Source: CAD feature listing. Evaluate the final solid. Frame: model axes, mm. Round coordinates to 2 decimals unless told otherwise and drop trailing zeros. Order: outer loops, then holes, each group sorted by start corner. A loop starts at its lowest first (then second) coordinate and runs counter-clockwise, first axis right, second up. Notation, with made-up numbers: (45.5, 76.25) - (49.5, 76.25) arc R21 ccw to (49.5, 109.25) - close; hole circle Ø10 at (1.25, 3). An arc over 180 degrees is marked (long way). Put each result on its own line as item: value. Start each with the question number.
1) Section A-A on z = 0. Output: boundary loops of the cut face in (x, y), then the cut area to 3 significant figures.
2) Line query: probe 1 along X at (y, z) = (9, 0); probe 2 along X at (y, z) = (17.75, 3); probe 3 along Z at (x, y) = (30.5, 2). Output: solid intervals per line, ascending. Write a range as [from, to].
3) Mould query, pull axis Z, two halves, no side actions, for faces 1 (the face through (46.99, 12.1, -22.15)), 2 (the face through (-4.88, 10.14, -1.08)), 3 (the face through (50, 12, 0)), 4 (the face through (-1, 12, 25)). Classes: +Z half, -Z half, draft (parallel to the pull), parting line (faces both ways), or undercut.
4) Section C-C on y = 11.25. Output: boundary loops of the cut face in (x, z), then the cut area to 3 significant figures.
5) Section B-B on x = 0. Output: boundary loops of the cut face in (y, z).
6) Contact query for a flat-ended pin moving along its axis: P1, Ø6, axis at x = 0, z = 0, coming from the +Y side. Output: stop coordinate, or through.
```python
from build123d import *

# Parameters (mm, degrees)
SKETCH1_W           = 100
SKETCH1_H           = 50
BOSS_EXTRUDE1_DEPTH = 20
SKETCH2_R           = 15
CUT_EXTRUDE1_DEPTH  = 20
FILLET1_R           = 10
CHAMFER1_SIZE       = 1
MOVE_FACE1_BY       = 10
FILLET2_R           = 5


with BuildPart() as part:
    # Sketch1 → Boss-Extrude1 (new body)
    with BuildSketch(Plane(origin=(0, 0, 0), x_dir=(1, 0, 0), z_dir=(0, 1, 0))):
        Rectangle(SKETCH1_W, SKETCH1_H)
    extrude(amount=BOSS_EXTRUDE1_DEPTH)

    # Sketch2 → Cut-Extrude1 (cut)
    with BuildSketch(Plane(origin=(0, 20, 0), x_dir=(1, 0, 0), z_dir=(0, 1, 0))):
        with Locations(Location((0, 0, 0), (0, 0, 270))):
            Circle(SKETCH2_R)
    extrude(amount=-CUT_EXTRUDE1_DEPTH, mode=Mode.SUBTRACT)

    # Fillet1
    fillet1_edges = [part.edges().sort_by_distance(p)[0] for p in [
        (50, 10, 25),
        (-50, 10, 25),
        (50, 10, -25),
    ]]
    fillet(fillet1_edges, radius=FILLET1_R)

    # Chamfer1
    chamfer1_edges = [part.edges().sort_by_distance(p)[0] for p in [
        (-50, 20, -5),
        (-5, 20, -25),
        (50, 20, 0),
        (0, 20, 25),
        (-47.071067812, 20, 22.071067812),
        (47.071067812, 20, 22.071067812),
        (47.071067812, 20, -22.071067812),
    ]]
    chamfer(chamfer1_edges, length=CHAMFER1_SIZE)

    # Move Face1: a curved face moved outward by 10.0
    add(Solid.thicken(part.faces().sort_by_distance((0, 10, -15))[0], MOVE_FACE1_BY))

    # Fillet2
    fillet2_edges = [part.edges().sort_by_distance(p)[0] for p in [
        (-5, 0, -25),
        (50, 0, 0),
        (0, 0, 25),
        (-47.071067812, 0, 22.071067812),
        (47.071067812, 0, 22.071067812),
        (47.071067812, 0, -22.071067812),
        (-50, 0, -5),
    ]]
    fillet(fillet2_edges, radius=FILLET2_R)


solid = part.part
```
Answer sheet:
1. outline: (-50, 5) arc R5 ccw to (-45, 0) - (-5, 0) - (-5, 20) - (-49, 20) - (-50, 19) - close; (5, 0) - (45, 0) arc R5 ccw to (50, 5) - (50, 19) - (49, 20) - (5, 20) - close
1. area: 1,790 mm^2
2. probe 1: [-50, -5], [5, 50]
2. probe 2: [-50, -4], [4, 50]
2. probe 3: [-24, 24]
3. face 1: -Z half
3. face 2: undercut
3. face 3: draft
3. face 4: +Z half
4. outline: (-50, -25) - (40, -25) arc R10 ccw to (50, -15) - (50, 15) arc R10 ccw to (40, 25) - (-40, 25) arc R10 ccw to (-50, 15) - close; hole circle Ø10 at (0, 0)
4. area: 4,860 mm^2
5. outline: (0, -20) arc R5 ccw to (5, -25) - (19, -25) - (20, -24) - (20, -5) - (0, -5) - close; (0, 5) - (20, 5) - (20, 24) - (19, 25) - (5, 25) arc R5 ccw to (0, 20) - close
6. P1: through
